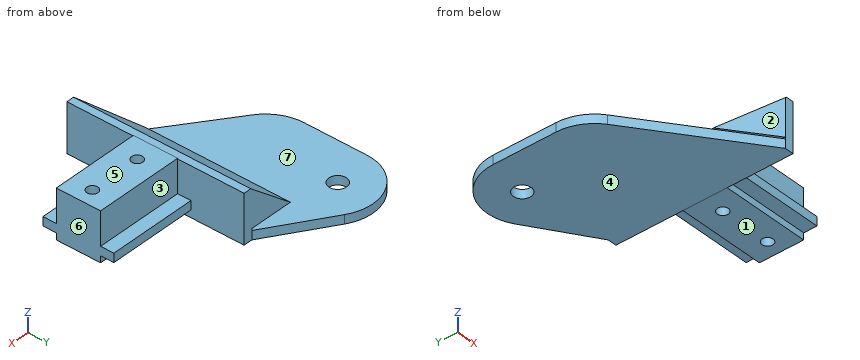
from build123d import *

# Parameters (mm, degrees)
SKETCH1_W                = 20
SKETCH1_H                = 10
BOSS_EXTRUDE1_DEPTH      = 11
BOSS_EXTRUDE2_DEPTH      = 3
BOSS_EXTRUDE2_DEPTH_BACK = 13
SKETCH2_W                = 20
SKETCH2_H                = 2
SKETCH3_W                = 11
SKETCH3_H                = 40
BOSS_EXTRUDE3_DEPTH      = 2
SKETCH5_W                = 2
SKETCH5_H                = 60
BOSS_EXTRUDE4_DEPTH      = 40
F_4_0MM_DOWEL_SLOT1_D    = 4
CUT_EXTRUDE1_DEPTH       = 40
CUT_EXTRUDE2_DEPTH       = 40
FILLET1_R                = 10
SKETCH11_W               = 53.631829023
SKETCH11_H               = 118.756200052
CUT_EXTRUDE3_DEPTH       = 40
FILLET2_R                = 10
SKETCH12_W               = 8.579575143
SKETCH12_H               = 40
BOSS_EXTRUDE5_DEPTH      = 10
CUT_EXTRUDE4_DEPTH       = 40
CUT_EXTRUDE5_DEPTH       = 40
F_2_5MM_DOWEL_SLOT1_D    = 2.5


with BuildPart() as part:
    # Sketch1 → Boss-Extrude1 (new body)
    with BuildSketch(Plane.XY):
        Rectangle(SKETCH1_W, SKETCH1_H)
    extrude(amount=BOSS_EXTRUDE1_DEPTH)

    # Sketch2 → Boss-Extrude2 (add, two sides: drawn at the far end of the back side and taken through both)
    with BuildSketch(Plane(origin=(0, 5, 0), x_dir=(1, 0, 0), z_dir=(0, 1, 0)).offset(-BOSS_EXTRUDE2_DEPTH_BACK)):
        with Locations((0, -2.5)):
            Rectangle(SKETCH2_W, SKETCH2_H)
    extrude(amount=BOSS_EXTRUDE2_DEPTH + BOSS_EXTRUDE2_DEPTH_BACK)

    # Sketch3 → Boss-Extrude3 (add)
    with BuildSketch(Plane.ZY.offset(10)):
        with Locations((5.357522791, 0)):
            Rectangle(SKETCH3_W, SKETCH3_H)
    extrude(amount=BOSS_EXTRUDE3_DEPTH)

    # Sketch5 → Boss-Extrude4 (add)
    with BuildSketch(Plane.ZY.offset(12)):
        with Locations((0.857522791, 10)):
            Rectangle(SKETCH5_W, SKETCH5_H)
    extrude(amount=BOSS_EXTRUDE4_DEPTH)

    # Ø4.0mm Dowel Slot1 (through all)
    with Locations(Plane(origin=(0, 0, -0.142477209), x_dir=(-1, 0, 0), z_dir=(0, 0, -1))):
        with Locations((32, 22)):
            Hole(F_4_0MM_DOWEL_SLOT1_D / 2)

    # Sketch9 → Cut-Extrude1 (cut)
    with BuildSketch(Plane(origin=(0, 0, -0.142477209), x_dir=(-1, 0, 0), z_dir=(0, 0, -1))):
        Polygon((12, 20), (31.113690538, 32.355186678), (52, 19.578846837), (52, 40), (12, 40), align=None)
    extrude(amount=-CUT_EXTRUDE1_DEPTH, mode=Mode.SUBTRACT)

    # Sketch10 → Cut-Extrude2 (cut)
    with BuildSketch(Plane.XY.offset(1.857522791)):
        Polygon((-12, -20), (-52, 9.223521766), (-52, -20), align=None)
    extrude(amount=-CUT_EXTRUDE2_DEPTH, mode=Mode.SUBTRACT)

    # Fillet1
    # the kernel refuses this fillet: 10 mm, written as the material it takes off along each edge
    with BuildSketch(Plane(origin=(-31.113690538, 32.355186678, -15.86551048), x_dir=(-0.8530548833247922, -0.5218212012133324, 0), z_dir=(0, 0, 1))) as fillet1_piece_1:
        with BuildLine():
            CenterArc((FILLET1_R * 0.628921330859, FILLET1_R), FILLET1_R, 205.666673807, 64.333326193)
            Line((-FILLET1_R * 0.27240777661, FILLET1_R * 0.566865101812), (0, 0))
            Line((0, 0), (FILLET1_R * 0.628921330859, 0))
        make_face()
    extrude(amount=33.446066543, mode=Mode.SUBTRACT)
    with BuildSketch(Plane(origin=(-52, 19.578846837, -14.156194501), x_dir=(0, -1, 0), z_dir=(0, 0, 1))) as fillet1_piece_2:
        with BuildLine():
            CenterArc((FILLET1_R * 0.560548691689, FILLET1_R), FILLET1_R, 211.454493545, 58.545506455)
            Line((-FILLET1_R * 0.292506191636, FILLET1_R * 0.478178798787), (0, 0))
            Line((0, 0), (FILLET1_R * 0.560548691689, 0))
        make_face()
    extrude(amount=30.027434584, mode=Mode.SUBTRACT)
    with BuildSketch(Plane(origin=(-52, 9.223521766, 14.554076611), x_dir=(0.8074608106822615, -0.5899212144111663, 0), z_dir=(0, 0, -1))) as fillet1_piece_3:
        with BuildLine():
            CenterArc((FILLET1_R * 0.507862152768, -FILLET1_R), FILLET1_R, 90, 53.848582464)
            Line((-FILLET1_R * 0.299598657914, -FILLET1_R * 0.410078785589), (0, 0))
            Line((0, 0), (FILLET1_R * 0.507862152768, 0))
        make_face()
    extrude(amount=27.393107638, mode=Mode.SUBTRACT)

    # Sketch11 → Cut-Extrude3 (cut)
    with BuildSketch(Plane.XY.offset(1.857522791)):
        with Locations((-67.994905589, 39.378925089)):
            Rectangle(SKETCH11_W, SKETCH11_H)
    extrude(amount=-CUT_EXTRUDE3_DEPTH, mode=Mode.SUBTRACT)

    # Fillet2
    # the kernel refuses this fillet: 10 mm, written as the material it takes off along each edge
    with BuildSketch(Plane(origin=(-41.178991077, 1.317822021, -12.839031028), x_dir=(0.8074608106822609, -0.589921214411167, 0), z_dir=(0, 0, 1))) as fillet2_piece_1:
        with BuildLine():
            CenterArc((FILLET2_R * 0.507862152768, FILLET2_R), FILLET2_R, 216.151417536, 53.848582464)
            Line((-FILLET2_R * 0.299598657914, FILLET2_R * 0.410078785589), (0, 0))
            Line((0, 0), (FILLET2_R * 0.507862152768, 0))
        make_face()
    extrude(amount=27.393107638, mode=Mode.SUBTRACT)
    with BuildSketch(Plane(origin=(-41.178991077, 26.198153502, 15.871240084), x_dir=(0, -1, 0), z_dir=(0, 0, -1))) as fillet2_piece_2:
        with BuildLine():
            CenterArc((FILLET2_R * 0.560548691689, -FILLET2_R), FILLET2_R, 90, 58.545506455)
            Line((-FILLET2_R * 0.292506191636, -FILLET2_R * 0.478178798787), (0, 0))
            Line((0, 0), (FILLET2_R * 0.560548691689, 0))
        make_face()
    extrude(amount=30.027434584, mode=Mode.SUBTRACT)

    # Sketch12 → Boss-Extrude5 (add)
    with BuildSketch(Plane.ZY.offset(12)):
        with Locations((6.56773522, 0)):
            Rectangle(SKETCH12_W, SKETCH12_H)
    extrude(amount=BOSS_EXTRUDE5_DEPTH)

    # Sketch13 → Cut-Extrude4 (cut)
    with BuildSketch(Plane.XZ.offset(20)):
        Polygon((-22, 2.277947648), (-11.725193368, 10.857522791), (-22, 10.857522791), align=None)
    extrude(amount=-CUT_EXTRUDE4_DEPTH, mode=Mode.SUBTRACT)

    # Sketch15 → Cut-Extrude5 (cut)
    with BuildSketch(Plane(origin=(0, 0, 2.277947648), x_dir=(-1, 0, 0), z_dir=(0, 0, -1))):
        Polygon((22, -20), (11.906976331, -20), (22, -12.461536252), align=None)
    extrude(amount=-CUT_EXTRUDE5_DEPTH, mode=Mode.SUBTRACT)

    # Ø2.5mm Dowel Slot1 (through all)
    with Locations(Plane.XY.offset(11)):
        with Locations((-5.250715138, 0), (6.374130199, 0)):
            Hole(F_2_5MM_DOWEL_SLOT1_D / 2)


solid = part.part
Can you work these out from the model? Positions are in its coordinate system, mm. Face numbers are marked on the shaded views. A direction names the side the tool comes from. Give positions to 0.01 mm unless a question says otherwise; leave off trailing zeros. Write each loop counter-clockwise with the first axis right and the second up, starting at its lowest first coordinate (ties: lowest second). Pieces come first, ordered by that corner, then holes. Notation, with made-up numbers: M 6.25,6 L 43.25,6 A16 ccw 43.25,13 Z; hole C 38,11.5 d6. An arc over 180 degrees is marked long. Answer in a Markdown table with one row per item. Add a question column.
Item 1: Imagine slicing it at A-A, the plane x = -32. Write out the boundary of the cut face in (y, z).
Item 2: Imagine slicing it at C-C, the plane x = 0. Write out the boundary of the cut face in (y, z), plus the area to 3 significant figures.
Item 3: We'd pull the mould along Z, two halves only. Please class the marked faces 5, 6 and 7: released by +Z, released by -Z, zero draft, split by the parting line, or undercut.
Item 4: For pin 1 Ø3.5 at (x, y) = (4, 7) entering from +Z; pin 2 Ø0.6 at (x, z) = (3, 3) entering from -Y; pin 3 Ø8 at (x, y) = (-3.5, -0.5) entering from -Z, each with a flat end and sliding along its axis, tell me the tip position at first contact or that it passes through.
Item 5: Imagine slicing it at D-D, the plane z = 6.75. Write out the boundary of the cut face in (x, y).
Item 6: On a 3-axis mill with a long thin cutter (end or side, diameter ignored), from which of +Z, -Z, +X, -X, +Y, -Y can I reach the whole of each face in a straight line? I mean the marked faces 1, 2, 3 and 4. Say none if no direction works.
Item 7: Please list where these lines run through material, in increasing order: L1, parallel to Z at x = 2.5, y = -2.5; L2, parallel to Y at x = 4, z = 9; L3, parallel to Z at x = -20.5, y = 19.5.
Item 8: Imagine slicing it at B-B, the plane y = 0. Write out the boundary of the cut face in (x, z).
Evaluation:
| question | item | result |
|---|---|---|
| 1 | outline | M -5.39,-0.14 L 20,-0.14 L 20,1.86 L -5.39,1.86 Z; M 24,-0.14 L 30.52,-0.14 L 30.52,1.86 L 24,1.86 Z |
| 2 | outline | M -8,1.5 L -5,1.5 L -5,0 L 5,0 L 5,1.5 L 8,1.5 L 8,3.5 L 5,3.5 L 5,11 L -5,11 L -5,3.5 L -8,3.5 Z |
| 2 | area | 122 mm² |
| 3 | face 5 | released by +Z |
| 3 | face 6 | zero draft |
| 3 | face 7 | undercut |
| 4 | pin 1 | stops at z = 3.5 |
| 4 | pin 2 | stops at y = -8 |
| 4 | pin 3 | stops at z = 0 |
| 5 | outline | M -16.64,-16.46 L -11.91,-20 L -10,-20 L -10,-5 L 10,-5 L 10,5 L -10,5 L -10,20 L -16.64,20 Z; hole C -5.25,0 d2.5; hole C 6.37,0 d2.5 |
| 6 | face 1 | -Z, +X, +Y, -Y |
| 6 | face 2 | +Z, -X, -Y |
| 6 | face 3 | +Z, +X, +Y |
| 6 | face 4 | -Z, +X, -X, +Y, -Y |
| 7 | L1 | z = 0 to 11 |
| 7 | L2 | y = -5 to 5 |
| 7 | L3 | z = -0.14 to 1.86, 2.28 to 3.53 |
| 8 | outline | M -38.87,-0.14 L -10,-0.14 L -10,0 L -6.5,0 L -6.5,11 L -10,11 L -10,10.86 L -11.73,10.86 L -22,2.28 L -12,2.28 L -12,1.86 L -38.87,1.86 Z; M -4,0 L 5.12,0 L 5.12,11 L -4,11 Z; M 7.62,0 L 10,0 L 10,11 L 7.62,11 Z |
